CAD build for the part. Positions are in the model's coordinates, mm. Face numbers are marked on the shaded views. A direction names the side the tool comes from. Round coordinates to 2 decimals unless told otherwise and drop trailing zeros. Loops run counter-clockwise (first coordinate to the right, second up) from the corner with the lowest first, then second, coordinate; pieces in that order, holes last. Notation, with made-up numbers: M -6,-0.5 L 20,-0.5 A24 ccw 20,36.5 Z; hole C -32,-36 d1. An arc over 180 degrees is marked long. Put each result on its own line as item: value. Start each with the question number.
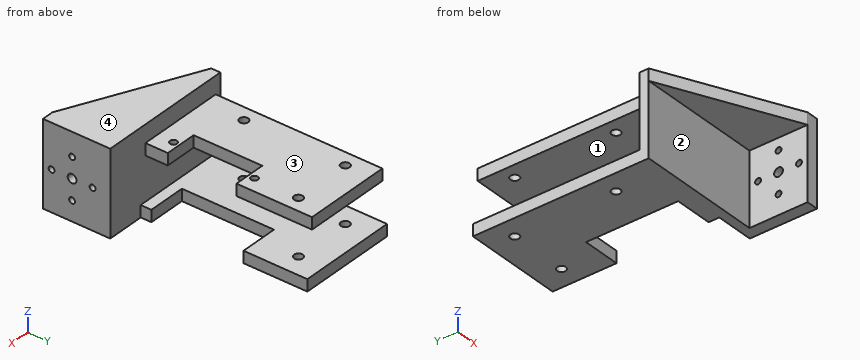
from build123d import *

# Parameters (mm, degrees)
SKETCH_1_R           = 1.5
SKETCH_1_R_2         = 1.2
EXTRUDE_1_DEPTH      = 4
SKETCH_2_W           = 19.899494937
SKETCH_2_H           = 19.899494937
SKETCH_2_R           = 1.5
EXTRUDE_2_DEPTH      = 4
EXTRUDE_3_DEPTH      = 15
EXTRUDE_3_DEPTH_BACK = 10
SKETCH_3_W           = 45
SKETCH_3_H           = 3.100505063
SKETCH_4_W           = 14.84
SKETCH_4_H           = 5
EXTRUDE_4_DEPTH      = 16
SKETCH_4_3_W         = 14.84
SKETCH_4_3_H         = 5
CUT_EXTRUDE_1_DEPTH  = 13
EXTRUDE_5_DEPTH      = 6
SKETCH_4_6_W         = 14.84
SKETCH_4_6_H         = 5
CUT_EXTRUDE_4_DEPTH  = 3
SKETCH_7_W           = 41
SKETCH_7_H           = 19.899494937
CUT_EXTRUDE_6_DEPTH  = 4
EXTRUDE_7_DEPTH      = 4
SKETCH_12_R          = 1.5
CUT_EXTRUDE_8_DEPTH  = 4
SKETCH_13_W          = 4
SKETCH_13_H          = 19.899494937
EXTRUDE_8_DEPTH      = 5.100505063
SKETCH_14_R          = 1.5
CUT_EXTRUDE_9_DEPTH  = 4
EXTRUDE_9_DEPTH      = 3.84
SKETCH_16_W          = 34
SKETCH_16_H          = 4
EXTRUDE_10_DEPTH     = 57
CUT_EXTRUDE_START    = -22.84
SKETCH_17_R          = 1.5
CUT_EXTRUDE_10_DEPTH = 22.84
SKETCH_18_W          = 2
SKETCH_18_H          = 3
EXTRUDE_11_DEPTH     = 3.100505063
SKETCH_19_W          = 24.84
SKETCH_19_H          = 3.100505063
EXTRUDE_12_DEPTH     = 2
EXTRUDE_13_DEPTH     = 4
SKETCH_21_W          = 13
SKETCH_21_H          = 31.5
CUT_EXTRUDE_11_DEPTH = 4
SKETCH_4_7_W         = 14.84
SKETCH_4_7_H         = 5
CUT_EXTRUDE_12_DEPTH = 16
SKETCH_22_W          = 2
SKETCH_22_H          = 3.100505063
EXTRUDE_14_DEPTH     = 1
SKETCH_23_R          = 1.5
EXTRUDE_15_DEPTH     = 4
SKETCH_24_R          = 1
CUT_EXTRUDE_13_DEPTH = 4


with BuildPart() as part:
    # Sketch 1 → Extrude 1 (new body)
    with BuildSketch(Plane.XY):
        Polygon((-15, -26), (-15, -54), (30, -54), (30, -31), (15, -31), (15, -26), (15, -23.333333333), (4, -23.333333333), (4, 0.166666667), (15, 0.166666667), (15, 26), (-15, 26), align=None)
        with Locations((-10, 17.333333333)):
            Circle(SKETCH_1_R, mode=Mode.SUBTRACT)
        with Locations((10, 17.333333333)):
            Circle(SKETCH_1_R, mode=Mode.SUBTRACT)
        with Locations((-10, -17.333333333)):
            Circle(SKETCH_1_R, mode=Mode.SUBTRACT)
        with Locations((10, 2.291666667)):
            Circle(SKETCH_1_R_2, mode=Mode.SUBTRACT)
        with Locations((10, -25.378333333)):
            Circle(SKETCH_1_R_2, mode=Mode.SUBTRACT)
    extrude(amount=EXTRUDE_1_DEPTH)

    # Sketch 2 → Extrude 2 (add)
    with BuildSketch(Plane(origin=(30, 0, 0), x_dir=(0, 0, -1), z_dir=(1, 0, 0))):
        with Locations((5.050252532, -44.050252531)):
            Rectangle(SKETCH_2_W, SKETCH_2_H)
        with Locations((0.100505063, -39.100505063)):
            Circle(SKETCH_2_R, mode=Mode.SUBTRACT)
        with Locations((10, -39.100505063)):
            Circle(SKETCH_2_R, mode=Mode.SUBTRACT)
        with Locations((0.100505063, -49)):
            Circle(SKETCH_2_R, mode=Mode.SUBTRACT)
        with Locations((10, -49)):
            Circle(SKETCH_2_R, mode=Mode.SUBTRACT)
    extrude(amount=-EXTRUDE_2_DEPTH)

    # Sketch 3 → Extrude 3 (add, two sides: drawn at the far end of the back side and taken through both)
    with BuildSketch(Plane(origin=(0, 0, 0), x_dir=(-1, 0, 0), z_dir=(0, 0, -1)).offset(-EXTRUDE_3_DEPTH_BACK)):
        with Locations((-7.5, -32.550252531)):
            Rectangle(SKETCH_3_W, SKETCH_3_H)
    extrude(amount=EXTRUDE_3_DEPTH + EXTRUDE_3_DEPTH_BACK)

    # Sketch 7 → Cut-Extrude 6 (cut)
    with BuildSketch(Plane(origin=(0, 0, 0), x_dir=(-1, 0, 0), z_dir=(0, 0, -1))):
        with Locations((-5.5, -44.050252531)):
            Rectangle(SKETCH_7_W, SKETCH_7_H)
    extrude(amount=-CUT_EXTRUDE_6_DEPTH, mode=Mode.SUBTRACT)

    # Sketch 10 → Extrude 7 (add)
    with BuildSketch(Plane.XY.offset(10)):
        Polygon((26, -54), (-15, -34.100505063), (26, -34.100505063), align=None)
    extrude(amount=-EXTRUDE_7_DEPTH)

    # Sketch 12 → Cut-Extrude 8 (cut)
    with BuildSketch(Plane(origin=(30, 0, 0), x_dir=(0, 0, -1), z_dir=(1, 0, 0))):
        with Locations(Location((5.050252532, -44.050252532, 0), (0, 0, 90))):
            Circle(SKETCH_12_R)
    extrude(amount=-CUT_EXTRUDE_8_DEPTH, mode=Mode.SUBTRACT)

    # Sketch 13 → Extrude 8 (add)
    with BuildSketch(Plane.XY.offset(4.899494937)):
        with Locations((28, -44.050252531)):
            Rectangle(SKETCH_13_W, SKETCH_13_H)
    extrude(amount=EXTRUDE_8_DEPTH)

    # Sketch 14 → Cut-Extrude 9 (cut)
    with BuildSketch(Plane(origin=(30, 0, 0), x_dir=(0, 0, -1), z_dir=(1, 0, 0))):
        with Locations((0.100505063, -49)):
            Circle(SKETCH_14_R)
        with Locations((0.100505063, -39.100505063)):
            Circle(SKETCH_14_R)
    extrude(amount=-CUT_EXTRUDE_9_DEPTH, mode=Mode.SUBTRACT)

    # Sketch 15 → Extrude 9 (add)
    with BuildSketch(Plane(origin=(0, 0, -15), x_dir=(-1, 0, 0), z_dir=(0, 0, -1))):
        Polygon((-30, -31), (-30, -54), (-26, -54), (-26, -34.100505063), (15, -34.100505063), (15, -31), align=None)
    extrude(amount=EXTRUDE_9_DEPTH)



with BuildPart() as body_2:
    # Sketch 4 → Extrude 4 (new body)
    with BuildSketch(Plane.ZY.offset(15)):
        with Locations((-7.42, -28.5)):
            Rectangle(SKETCH_4_W, SKETCH_4_H)
    extrude(amount=-EXTRUDE_4_DEPTH)

    # Sketch 4_3 → Cut-Extrude 1 (cut)
    with BuildSketch(Plane.ZY.offset(15)):
        with Locations((-7.42, -28.5)):
            Rectangle(SKETCH_4_3_W, SKETCH_4_3_H)
    extrude(amount=-CUT_EXTRUDE_1_DEPTH, mode=Mode.SUBTRACT)


with BuildPart() as body_3:
    # Sketch 4 → Extrude 5 (new body)
    with BuildSketch(Plane.ZY.offset(15)):
        with Locations((-7.42, -28.5)):
            Rectangle(SKETCH_4_W, SKETCH_4_H)
    extrude(amount=-EXTRUDE_5_DEPTH)

    # Sketch 4_6 → Cut-Extrude 4 (cut)
    with BuildSketch(Plane.ZY.offset(15)):
        with Locations((-7.42, -28.5)):
            Rectangle(SKETCH_4_6_W, SKETCH_4_6_H)
    extrude(amount=-CUT_EXTRUDE_4_DEPTH, mode=Mode.SUBTRACT)


with BuildPart() as part_1:
    add(part.part)

    add(body_2.part)  # Extrude 10 merges body 2

    add(body_3.part)  # Extrude 10 merges body 3
    # Sketch 16 → Extrude 10 (add)
    with BuildSketch(Plane(origin=(0, -31, 0), x_dir=(1, 0, 0), z_dir=(0, 1, 0))):
        with Locations((0, 16.84)):
            Rectangle(SKETCH_16_W, SKETCH_16_H)
    extrude(amount=EXTRUDE_10_DEPTH)

    # Sketch 17 → Cut-Extrude 10 (cut)
    with BuildSketch(Plane.XY.offset(4).offset(CUT_EXTRUDE_START)):
        with Locations((-10, -17.333333333)):
            Circle(SKETCH_17_R)
        with Locations((-10, 17.333333333)):
            Circle(SKETCH_17_R)
        with Locations((10, 17.333333333)):
            Circle(SKETCH_17_R)
    extrude(amount=CUT_EXTRUDE_10_DEPTH, mode=Mode.SUBTRACT)

    # Sketch 18 → Extrude 11 (add)
    with BuildSketch(Plane.XZ.offset(31)):
        with Locations((-16, -16.34)):
            Rectangle(SKETCH_18_W, SKETCH_18_H)
    extrude(amount=EXTRUDE_11_DEPTH)

    # Sketch 19 → Extrude 12 (add)
    with BuildSketch(Plane.ZY.offset(15)):
        with Locations((-2.42, -32.550252531)):
            Rectangle(SKETCH_19_W, SKETCH_19_H)
    extrude(amount=EXTRUDE_12_DEPTH)

    # Sketch 20 → Extrude 13 (add)
    with BuildSketch(Plane.XY.offset(10)):
        Polygon((26, -54), (-17, -34.100505063), (26, -34.100505063), align=None)
    extrude(amount=-EXTRUDE_13_DEPTH)

    # Sketch 21 → Cut-Extrude 11 (cut)
    with BuildSketch(Plane.XY.offset(-14.84)):
        with Locations((10.5, -11.583333333)):
            Rectangle(SKETCH_21_W, SKETCH_21_H)
    extrude(amount=-CUT_EXTRUDE_11_DEPTH, mode=Mode.SUBTRACT)

    # Sketch 4_7 → Cut-Extrude 12 (cut)
    with BuildSketch(Plane.ZY.offset(15)):
        with Locations((-7.42, -28.5)):
            Rectangle(SKETCH_4_7_W, SKETCH_4_7_H)
    extrude(amount=-CUT_EXTRUDE_12_DEPTH, mode=Mode.SUBTRACT)

    # Sketch 22 → Extrude 14 (add)
    with BuildSketch(Plane(origin=(0, 0, -17.84), x_dir=(-1, 0, 0), z_dir=(0, 0, -1))):
        with Locations((16, -32.550252531)):
            Rectangle(SKETCH_22_W, SKETCH_22_H)
    extrude(amount=EXTRUDE_14_DEPTH)

    # Sketch 23 → Extrude 15 (add)
    with BuildSketch(Plane(origin=(30, 0, 0), x_dir=(0, 0, -1), z_dir=(1, 0, 0))):
        with Locations((0.100505063, -49)):
            Circle(SKETCH_23_R)
        with Locations((0.100505063, -39.100505063)):
            Circle(SKETCH_23_R)
        with Locations((10, -49)):
            Circle(SKETCH_23_R)
        with Locations((10, -39.100505063)):
            Circle(SKETCH_23_R)
    extrude(amount=-EXTRUDE_15_DEPTH)

    # Sketch 24 → Cut-Extrude 13 (cut)
    with BuildSketch(Plane(origin=(30, 0, 0), x_dir=(0, 0, -1), z_dir=(1, 0, 0))):
        with Locations(Location((-1.949747468, -44.050252532, 0), (0, 0, 90))):
            Circle(SKETCH_24_R)
        with Locations(Location((12.050252532, -44.050252532, 0), (0, 0, 90))):
            Circle(SKETCH_24_R)
        with Locations(Location((5.050252532, -37.050252532, 0), (0, 0, 90))):
            Circle(SKETCH_24_R)
        with Locations(Location((5.050252532, -51.050252532, 0), (0, 0, 90))):
            Circle(SKETCH_24_R)
    extrude(amount=-CUT_EXTRUDE_13_DEPTH, mode=Mode.SUBTRACT)


solid = part_1.part
(1) Drill centre lines: line 1 along Y through (x, z) = (-10, -16.6); line 2 along Y through (x, z) = (10, 2); line 3 along Z through (x, y) = (12, 14). Where is each one in solid material? Low to high.
(2) Cut at A-A on y = 14.5. List the corners of the cut face in (x, z), and give its area (3 significant figures).
(3) Cut at C-C on y = -6. List the corners of the cut face in (x, z), and give its area (3 significant figures).
(4) Tool access for the marked faces 1, 2, 3 and 4: list every direction of +Z, -Z, +X, -X, +Y, -Y with a clear straight run to the whole face (end or side of a thin tool).
(5) Flat gauge pins, fed straight in: pin 1 Ø4.5 at (y, z) = (-11, -16.5) entering from +X; pin 2 Ø10 at (x, z) = (5, 7) entering from -Y; pin 3 Ø2 at (x, y) = (14.5, -24.5) entering from +Z. Where does each tip first touch, or does it go through?
(6) Cut at D-D on z = -9.75. List the corners of the cut face in (x, y), and give its area (3 significant figures).
(7) Cut at B-B on x = -10. List the corners of the cut face in (y, z).
Taken from the geometry:
1. line 1: -34.1 to -18.83, -15.83 to 15.83, 18.83 to 26
1. line 2: -34.1 to -26.58, -24.18 to -23.33, 0.17 to 1.09, 3.49 to 15.83, 18.83 to 26
1. line 3: -18.84 to -14.84, 0 to 4
2. outline: M -17,-18.84 L 17,-18.84 L 17,-14.84 L -17,-14.84 Z; M -15,0 L 15,0 L 15,4 L -15,4 Z
2. area: 256 mm2
3. outline: M -17,-18.84 L 4,-18.84 L 4,-14.84 L -17,-14.84 Z; M -15,0 L 4,0 L 4,4 L -15,4 Z
3. area: 160 mm2
4. face 1: +X, -X, +Y
4. face 2: -Z, -X, -Y
4. face 3: +Z, +X, -X, +Y
4. face 4: +Z, +X, -X, +Y, -Y
5. pin 1: x = 4
5. pin 2: y = -46.6
5. pin 3: z = 4
6. outline: M -17,-34.1 L 26,-34.1 L 26,-54 L 30,-54 L 30,-31 L -17,-31 Z
6. area: 225 mm2
7. outline: M -37.34,6 L -34.1,6 L -34.1,-18.84 L -18.83,-18.84 L -18.83,-14.84 L -31,-14.84 L -31,0 L -18.83,0 L -18.83,4 L -31,4 L -31,10 L -37.34,10 Z; M -15.83,-18.84 L 15.83,-18.84 L 15.83,-14.84 L -15.83,-14.84 Z; M -15.83,0 L 15.83,0 L 15.83,4 L -15.83,4 Z; M 18.83,-18.84 L 26,-18.84 L 26,-14.84 L 18.83,-14.84 Z; M 18.83,0 L 26,0 L 26,4 L 18.83,4 Z
